For this review, take the finished solid that the model builds, in its own axes (mm). Face numbers are marked on the shaded views. A direction names the side the tool comes from. Give positions to 0.01 mm unless a question says otherwise; leave off trailing zeros. Loops run counter-clockwise (first coordinate to the right, second up) from the corner with the lowest first, then second, coordinate; pieces in that order, holes last.
```python
from build123d import *

# Parameters (mm, degrees)
BOSS_EXTRUDE1_DEPTH = 3
FILLET1_R           = 1
SKETCH20_W          = 15.9
SKETCH20_H          = 7.95
BOSS_EXTRUDE2_DEPTH = 3
SHELL1_T            = -1.2
SKETCH21_W          = 7
SKETCH21_H          = 2
BOSS_EXTRUDE4_DEPTH = 7
CUT_EXTRUDE1_DEPTH  = 25.097211976
SKETCH23_R          = 2.4
SKETCH23_R_2        = 1.4
BOSS_EXTRUDE5_DEPTH = 1.8


with BuildPart() as part:
    # Sketch1 → Boss-Extrude1 (new body)
    with BuildSketch(Plane(origin=(0, 0, 0), x_dir=(1, 0, 0), z_dir=(0, 1, 0))):
        with BuildLine():
            Line((-12.5, -7.5), (12.5, -7.5))
            ThreePointArc((12.5, -7.5), (20, 0), (12.5, 7.5))
            Line((12.5, 7.5), (-12.5, 7.5))
            ThreePointArc((-12.5, 7.5), (-20, 0), (-12.5, -7.5))
        make_face()
    extrude(amount=BOSS_EXTRUDE1_DEPTH)

    # Fillet1
    fillet1_edges = [part.edges().sort_by_distance(p)[0] for p in [
        (-20, 3, 0),
        (0, 3, 7.5),
        (20, 3, 0),
        (0, 0, 7.5),
        (-20, 0, 0),
        (0, 0, -7.5),
        (20, 0, 0),
        (0, 3, -7.5),
    ]]
    fillet(fillet1_edges, radius=FILLET1_R)

    # Sketch20 → Boss-Extrude2 (add)
    with BuildSketch(Plane.XZ):
        Rectangle(SKETCH20_W, SKETCH20_H)
    extrude(amount=BOSS_EXTRUDE2_DEPTH)

    # Shell1
    shell1_openings = [part.faces().sort_by_distance(p)[0] for p in [
        (0, -3, 0),
    ]]
    offset(amount=SHELL1_T, openings=shell1_openings, kind=Kind.INTERSECTION)

    # Sketch21 → Boss-Extrude4 (add)
    with BuildSketch(Plane.XZ):
        with Locations((11.45, -2.975)):
            Rectangle(SKETCH21_W, SKETCH21_H)
        with Locations((11.45, 2.975)):
            Rectangle(SKETCH21_W, SKETCH21_H)
    boss_extrude4 = extrude(amount=BOSS_EXTRUDE4_DEPTH)

    # Sketch22 → Cut-Extrude1 (cut, through all)
    with BuildSketch(Plane.XY.offset(3.975)):
        with BuildLine():
            Line((11.95, -7), (10.95, -7))
            Line((10.95, -7), (10.95, -5.748331477))
            ThreePointArc((10.95, -5.748331477), (11.45, -4.1), (11.95, -5.748331477))
            Line((11.95, -5.748331477), (11.95, -7))
        make_face()
    cut_extrude1 = extrude(amount=-CUT_EXTRUDE1_DEPTH, mode=Mode.SUBTRACT)

    # Mirror1: Boss-Extrude4, Cut-Extrude1 across plane
    add(boss_extrude4.mirror(Plane(origin=(0, 0, 0), x_dir=(0, 0, 1), z_dir=(1, 0, 0))))
    add(cut_extrude1.mirror(Plane(origin=(0, 0, 0), x_dir=(0, 0, 1), z_dir=(1, 0, 0))), mode=Mode.SUBTRACT)

    # Sketch23 → Boss-Extrude5 (add)
    with BuildSketch(Plane(origin=(0, 3, 0), x_dir=(1, 0, 0), z_dir=(0, 1, 0))):
        with Locations(Location((-4, 0, 0), (0, 0, 270))):
            Circle(SKETCH23_R)
        with Locations(Location((-4, 0, 0), (0, 0, 270))):
            Circle(SKETCH23_R_2, mode=Mode.SUBTRACT)
    boss_extrude5 = extrude(amount=BOSS_EXTRUDE5_DEPTH)

    # Mirror2: Boss-Extrude5 across plane
    add(boss_extrude5.mirror(Plane(origin=(0, 0, 0), x_dir=(0, 0, 1), z_dir=(1, 0, 0))))


solid = part.part
```
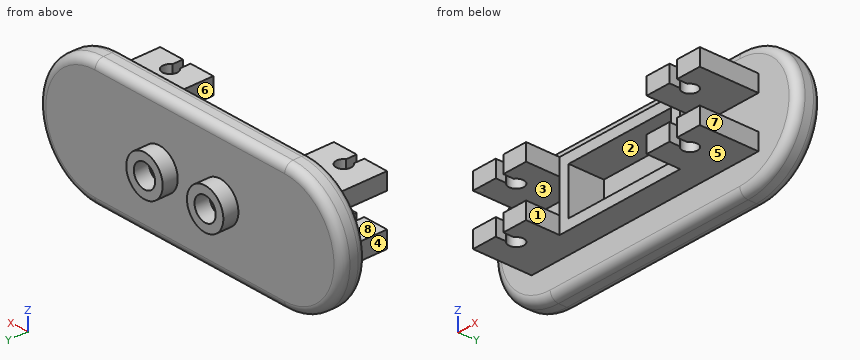
Q1. For pin 1 Ø6 at (y, z) = (-4, -4.5) entering from -X; pin 2 Ø3.5 at (x, y) = (-1, -0.5) entering from -Z; pin 3 Ø3 at (x, y) = (15.5, -1) entering from +Z; pin 4 Ø2 at (x, y) = (11.45, -5) entering from -Z (3 decimals), all flat-tipped, find the tip position at first contact; note any pin that passes through.
Answers:
pin 1: stops at x = -14.95
pin 2: stops at z = -7.5
pin 3: stops at z = 6.87
pin 4: stops at z = -3.975
Q2. Machinability: for the marked faces 1, 2, 3, 4 and 5, which of the approach directions +Z, -Z, +X, -X, +Y, -Y give a long, thin tool a straight path to every point of the face, cutting with its end or side? Answer none if there is none.
Answers:
face 1: +Z, -Z, -Y
face 2: -Y
face 3: -X, -Y
face 4: +Z, -Z, -X, -Y
face 5: -Z, +X, -X, -Y
Q3. For probe 1 along X at (y, z) = (4.1, 0); probe 2 along X at (y, z) = (-5, -3.1); probe 3 along Y at (x, z) = (-11.5, 0), list the stretches that pass through material, from the lowest coordinate up.
Answers:
probe 1: x = -6.4 to -5.4, -2.6 to -1.6, 1.6 to 2.6, 5.4 to 6.4
probe 2: x = -14.95 to -12.35, -10.55 to -7.95, 7.95 to 10.55, 12.35 to 14.95
probe 3: y = 0 to 1.2, 1.8 to 3
Q4. Consider section B-B on x = -11.45. Give the boundary of the cut face in (y, z) (3 decimals).
Answers:
outline: (-4.1, -3.975) - (0, -3.975) - (0, -6.5) arc R1 ccw to (1, -7.5) - (2, -7.5) arc R1 ccw to (3, -6.5) - (3, 6.5) arc R1 ccw to (2, 7.5) - (1, 7.5) arc R1 ccw to (0, 6.5) - (0, 3.975) - (-4.1, 3.975) - (-4.1, 1.975) - (0, 1.975) - (0, -1.975) - (-4.1, -1.975) - close; hole (1.2, -6.3) - (1.8, -6.3) - (1.8, 6.3) - (1.2, 6.3) - close
Q5. Mouldability with a two-part tool opening along X and no side actions: class the marked faces 6, 7 and 8 as +X half, -X half, draft (parallel to the pull), parting line (faces both ways), or undercut.
Answers:
face 6: undercut
face 7: +X half
face 8: draft
Q6. Consider section D-D on x = 1. Give the boundary of the cut face in (y, z) (3 decimals), plus the area to 3 significant figures.
Answers:
outline: (-3, -3.975) - (0, -3.975) - (0, -6.5) arc R1 ccw to (1, -7.5) - (2, -7.5) arc R1 ccw to (3, -6.5) - (3, 6.5) arc R1 ccw to (2, 7.5) - (1, 7.5) arc R1 ccw to (0, 6.5) - (0, 3.975) - (-3, 3.975) - (-3, 2.775) - (1.2, 2.775) - (1.2, 6.3) - (1.8, 6.3) - (1.8, -6.3) - (1.2, -6.3) - (1.2, -2.775) - (-3, -2.775) - close
area: 37.1 mm2
Q7. Consider section A-A on y = -5. Count the separate pieces of the cut face and the enclosed holes in it, plus the area to 3 significant figures.
Answers:
separate pieces: 8
enclosed holes: 0
area: 41.6 mm2
Q8. Consider section C-C on x = -4. Give the boundary of the cut face in (y, z) (3 decimals), plus the area to 3 significant figures.
Answers:
outline: (-3, -3.975) - (0, -3.975) - (0, -6.5) arc R1 ccw to (1, -7.5) - (2, -7.5) arc R1 ccw to (3, -6.5) - (3, -2.4) - (4.8, -2.4) - (4.8, -1.4) - (3, -1.4) - (3, 1.4) - (4.8, 1.4) - (4.8, 2.4) - (3, 2.4) - (3, 6.5) arc R1 ccw to (2, 7.5) - (1, 7.5) arc R1 ccw to (0, 6.5) - (0, 3.975) - (-3, 3.975) - (-3, 2.775) - (1.2, 2.775) - (1.2, 6.3) - (1.8, 6.3) - (1.8, -6.3) - (1.2, -6.3) - (1.2, -2.775) - (-3, -2.775) - close
area: 40.7 mm2
